Geometry check sheet. Reference: the model listing, model coordinates, mm. Round coordinates to 2 decimals unless told otherwise and drop trailing zeros. Order: outer loops, then holes, each group sorted by start corner. A loop starts at its lowest first (then second) coordinate and runs counter-clockwise, first axis right, second up.
Autodesk Inventor part; units mm, degrees
ref_plane "YZ Plane" through (0, 0, 0) normal (1, 0, 0) x (0, 1, 0)
ref_plane "XZ Plane" through (0, 0, 0) normal (0, 1, 0) x (-1, 0, 0)
ref_plane "XY Plane" through (0, 0, 0) normal (0, 0, 1) x (1, 0, 0)
sketch "Sketch1" plane through (0, 0, 0) normal (0, 1, 0) x (-1, 0, 0)
  line L0 (-97.5, -62.5) -> (97.5, -62.5)
  line L1 (97.5, 62.5) -> (-97.5, 62.5)
  line L2 (-97.5, 62.5) -> (-97.5, -62.5)
  line L3 (-97.5, -62.5) -> (97.5, 62.5) construction
  line L4 (97.5, -62.5) -> (-97.5, 62.5) construction
  line L5 (97.5, 20) -> (112.525, 20)
  line L6 (127.475, 21.2237) -> (127.475, -18.7763)
  line L7 (112.525, -17.5526) -> (97.5, -17.5526)
  line L8 (97.5, -62.5) -> (97.5, -17.5526)
  line L9 (97.5, 20) -> (97.5, 62.5)
  line L10 (112.525, 20) -> (112.525, 61)
  line L11 (127.475, 61) -> (127.475, 21.2237)
  line L12 (127.475, 1.2237) -> (97.475, 1.2237) construction
  line L13 (112.525, -17.5526) -> (112.525, -58.5526)
  line L14 (127.475, -58.5526) -> (127.475, -18.7763)
  line L15 (119.975, 61) -> (121.775, 61) construction
  line L16 (121.775, 61) -> (121.775, 59)
  line L17 (118.225, 61) -> (118.225, 59)
  line L18 (121.775, 59) -> (125.775, 59)
  line L19 (125.775, 59) -> (125.775, 56.5)
  line L20 (125.775, 56.5) -> (121.775, 56.5)
  line L21 (121.775, 61) -> (121.775, 53) construction
  line L22 (119.975, 61) -> (119.975, 52.3078) construction
  line L23 (118.225, 59) -> (114.175, 59)
  line L24 (114.175, 59) -> (114.175, 56.5)
  line L25 (114.175, 56.5) -> (118.175, 56.5)
  line L26 (118.175, 56.5) -> (118.175, 53.5)
  line L27 (112.525, 61) -> (118.225, 61)
  line L28 (127.475, 61) -> (121.775, 61)
  line L29 (119.975, -58.5526) -> (121.775, -58.5526) construction
  line L30 (112.525, -58.5526) -> (118.225, -58.5526)
  line L31 (127.475, -58.5526) -> (121.775, -58.5526)
  line L32 (121.775, 56.5) -> (121.775, 47.5)
  line L33 (118.175, 53.5) -> (118.175, 47.5)
  line L34 (118.175, 47.5) -> (121.775, 47.5)
  line L35 (119.975, -58.5526) -> (121.775, -58.5526) construction
  line L36 (121.775, -58.5526) -> (121.775, -56.5526)
  line L37 (118.225, -58.5526) -> (118.225, -56.5526)
  line L38 (121.775, -56.5526) -> (125.775, -56.5526)
  line L39 (125.775, -56.5526) -> (125.775, -54.0526)
  line L40 (125.775, -54.0526) -> (121.775, -54.0526)
  line L41 (121.775, -58.5526) -> (121.775, -50.5526) construction
  line L42 (119.975, -58.5526) -> (119.975, -49.8604) construction
  line L43 (114.175, -54.0526) -> (118.175, -54.0526)
  line L44 (114.175, -56.5526) -> (114.175, -54.0526)
  line L45 (118.225, -56.5526) -> (114.175, -56.5526)
  line L46 (118.175, -54.0526) -> (118.175, -51.0526)
  line L47 (112.525, -58.5526) -> (118.225, -58.5526)
  line L48 (127.475, -58.5526) -> (121.775, -58.5526)
  line L49 (121.775, -54.0526) -> (121.775, -45.0526)
  line L50 (118.175, -51.0526) -> (118.175, -45.0526)
  line L51 (118.175, -45.0526) -> (121.775, -45.0526)
  line L52 (127.475, 61) -> (127.475, 79) construction
  line L53 (-97.5, 0) -> (-67.5, 0) construction
  line L54 (-67.5, 62.5) -> (-67.5, -62.5) construction
  line L55 (127.475, 79) -> (-67.5, 0) construction
  line L56 (127.475, -58.5526) -> (127.475, -76.5526) construction
  line L57 (127.475, -76.5526) -> (-67.5, 0) construction
  line L58 (-97.5, 62.5) -> (-117.5, 62.5)
  line L59 (-117.5, 62.5) -> (-117.5, -62.5)
  line L60 (-117.5, -62.5) -> (-97.5, -62.5)
  line L61 (-97.5, -62.5) -> (-97.5, 62.5)
  line L62 (-67.5, 0) -> (-47.5, 0) construction
  circle A0 centre (-47.5, 0) radius 1.6
  line L63 (-67.5, 0) -> (-87.5, 0) construction
  circle A1 centre (-87.5, 0) radius 1.6
  point P0 (0, 0)
  point P1 (121.775, 53.5)
  point P2 (121.775, -51.0526)
  point P3 (-97.5, -62.5)
  dimension "d0" = 195
  dimension "d1" = 125
  dimension "d3" = 30
  dimension "d4" = 40
  dimension "d5" = 15
  dimension "d6" = 41
  dimension "d11" = 7.5
  dimension "d12" = 1.8
  dimension "d13" = 1.75
  dimension "d14" = 2
  dimension "d15" = 2
  dimension "d17" = 2.5
  dimension "d18" = 8
  dimension "d19" = 3
  dimension "d21" = 30
  dimension "d22" = 8.6922
  dimension "d23" = 1.5
  dimension "d25" = 4
  dimension "d26" = 13.25
  dimension "d27" = 9
  dimension "d28" = 18
  dimension "d29" = 30
  dimension "d30" = 18
  dimension "d35" = 20
  dimension "d36" = 125
  dimension "d41" = 20
  dimension "d42" = 3.2
  dimension "d43" = 20
  dimension "d47" = 3.2
extrude "Extrusion1" add sketch "Sketch1" along normal blind 3.25 contours L2 L1 L9 L5 L10 L27 L17 L23 L24 L25 L26 L33 L34 L32 L20 L19 L18 L16 L28 L11 L6 L14 L31 L36 L38 L39 L40 L49 L51 L50 L46 L43 L44 L45 L37 L30 L13 L7 L8 L0 | A0 | A1
sketch "Sketch2" plane through (0, 3.25, 0) normal (0, 1, 0) x (1, 0, 0)
  line L0 (-127.475, 58.5526) -> (-127.475, -61) construction
  line L1 (-127.475, 0) -> (-59.475, 0) construction
  circle A0 centre (-59.475, 0) radius 5
  point P0 (0, 0)
  dimension "d31" = 68
  dimension "d32" = 10
extrude "Extrusion2" cut sketch "Sketch2" against normal blind 10
sketch "Sketch3" plane through (97.5, 0, 62.5) normal (1, 0, 0) x (0, 0, -1)
  line L0 (125, 0) -> (80.0526, 0)
  line L1 (0, 3.25) -> (125, 3.25)
  line L2 (125, 3.25) -> (125, 0)
  line L3 (125, 0) -> (0, 0)
  line L4 (0, 0) -> (0, 3.25)
  point P0 (62.5, 0)
extrude "Extrusion4" add sketch "Sketch3" along normal blind 30
extrude "Extrusion5" cut sketch "Sketch1" along normal blind 4 contours A0 | A1
properties part number "suelo_imp"
(1) Material ranges on line 1 (X direction, y = 1.4, z = 0) (3 decimals); line 2 (X direction, y = 2.35, z = -55.5) (3 decimals); line 3 (X direction, y = 0.2, z = 53) (3 decimals), recorded low to high.
Returned:
line 1: x = -127.475 to -64.475, -54.475 to 45.9, 49.1 to 85.9, 89.1 to 127.5
line 2: x = -127.475 to -125.775, -114.175 to -112.525, -97.5 to 127.5
line 3: x = -127.475 to -121.775, -118.175 to -112.525, -97.5 to 127.5
(2) Sectioned sample at B-B, the plane y = 1.45. Give the number of separate pieces and of enclosed holes in the cut face, and give its area (3 significant figures).
Returned:
separate pieces: 1
enclosed holes: 3
area: 30,200 mm2
(3) Draft check along Z on faces 1 (the flat face through (-2, 3.25, 1)), 2 (the cylindrical face through (-64.47, 1.65, -0.22)). Enter one of: released by +Z, released by -Z, zero draft, split by the parting line, or undercut.
Returned:
face 1: zero draft
face 2: undercut
(4) Sectioned sample at A-A, the plane z = -30.5. Record the cut outline in (x, y) (3 decimals), and give its area (3 significant figures).
Returned:
outline: (-127.475, 0) - (-112.525, 0) - (-112.525, 3.25) - (-127.475, 3.25) - close; (-97.5, 0) - (127.5, 0) - (127.5, 3.25) - (-97.5, 3.25) - close
area: 780 mm2
(5) Depth check by flat-ended pin: P1, Ø1.6, axis at x = -119.5, y = 2, coming from the +Z side; P2, Ø1.6, axis at x = -124, y = 1.5, coming from the -Z side; P3, Ø1, axis at x = -116, y = 2.5, coming from the +Z side. Enter the tip coordinate at first touch or a pass-through.
Returned:
P1: stops at z = 47.5
P2: stops at z = -58.55
P3: stops at z = 61
